Work out the finished part from the listing and answer in its coordinate system (mm). Face numbers are marked on the shaded views. A direction names the side the tool comes from. Give positions to 0.01 mm unless a question says otherwise; leave off trailing zeros. Write each loop counter-clockwise with the first axis right and the second up, starting at its lowest first coordinate (ties: lowest second). Pieces come first, ordered by that corner, then holes. Notation, with made-up numbers: (7.25, 80.5) -> (32.25, 80.5) arc R19 ccw to (32.25, 89.5) -> close; hole circle Ø9 at (-13, 29). An arc over 180 degrees is marked (long way). Use a Markdown table: item, result. Add a question column.
Q1. Section A-A, the plane z = -5.5 is taken. Give the vertices of the cut face in (x, y), plus the area to 3 significant figures.
Q2. For the marked faces 5, 6 and 7, determine the directions among +Z, -Z, +X, -X, +Y, -Y from which every point of the face is accessible in a straight line to the end or side of a thin tool.
Q3. For a pull along X with two mould halves and no side action, classify the marked faces 1, 2, 3 and 4 as pulls with the +X half, pulls with the -X half, needs draft (parallel to the pull), parting line crosses it, or undercut.
Q4. Section D-D, the plane z = 1.5 is taken. Give the vertices of the cut face in (x, y), plus the area to 3 significant figures.
Q5. Section B-B, the plane x = -1.5 is taken. Give the vertices of the cut face in (y, z).
Q6. Consider line 1 (Z direction, x = 0, y = -1.75); line 2 (X direction, y = -5, z = 0). Determine where each line is inside the solid, lowest interval first.
Q7. Each of these flat-tipped pins is pushed along its axis until it touches: pin 1 Ø4 at (x, z) = (4, 3) entering from -Y; pin 2 Ø1 at (x, y) = (0, -4) entering from +Z. Where does it stop, or does it pass through?
Q8. Section C-C, the plane y = -5.75 is taken. Give the vertices of the cut face in (x, z).
from build123d import *
from build123d import SkipClean  # not in build123d's __all__

# Parameters (mm, degrees)
F1_DEPTH = 2.5
F4_SIZE  = 0.7
F3_W     = 2.5
F3_H     = 1.2


with BuildPart() as f1:
    # F0 (on Front) → F1 (new body)
    with BuildSketch(Plane.XZ):
        with BuildLine():
            Line((0, 4), (-9, 4))
            Line((-9, 4), (-9, 3.3))
            Line((-9, 3.3), (-8.3, 3.3))
            Line((-8.3, 3.3), (-8.3, 2.6))
            Line((-8.3, 2.6), (-9, 2.6))
            Line((-9, 2.6), (-9, 1.9))
            Line((-9, 1.9), (-8.3, 1.9))
            Line((-8.3, 1.9), (-8.3, 1.2))
            Line((-8.3, 1.2), (-9, 1.2))
            Line((-9, 1.2), (-9, 0.5))
            Line((-9, 0.5), (-8.3, 0.5))
            Line((-8.3, 0.5), (-8.3, -0.2))
            Line((-8.3, -0.2), (-9, -0.2))
            Line((-9, -0.2), (-9, -7))
            Line((-9, -7), (-7.8, -7))
            Line((-7.8, -7), (-7.8, -2.900873477))
            add(Edge.make_bspline(
                [(-7.8, -2.900873477), (-7.8, -1.685574969), (-7.1826716424, -0.1281665724), (-4.9759016066, 0.6847768295), (-3.5267368498, -0.4819738014), (-3.0814464759, -1.4369020899)],
                knots=[0, 0, 0, 0, 0.3572792207, 0.6508868549, 1, 1, 1, 1], degree=3))
            ThreePointArc((-3.0814464759, -1.4369020899), (-1.8268186684, -2.8675309158), (0, -3.4))
            Line((0, -3.4), (0, -2.4))
            ThreePointArc((0, -2.4), (-2.4, 0), (0, 2.4))
            Line((0, 2.4), (0, 4))
        make_face()
    extrude(amount=F1_DEPTH)

    # F2: F1 across plane


with BuildPart() as f1_1:
    add(f1.part, clean=False)
    with SkipClean():  # cleaning this boolean's faces spoils the solid; the shape is the same uncleaned
        add(f1.part.mirror(Plane.YZ), clean=False)

    # F4
    f4_edges = [f1_1.edges().sort_by_distance(p)[0] for p in [
        (-9, -2.5, -3.6),
        (9, -2.5, -3.6),
        (-9, -2.5, 3.65),
        (-9, -2.5, 2.25),
        (-9, -2.5, 0.85),
        (9, -2.5, 3.65),
        (9, -2.5, 2.25),
        (9, -2.5, 0.85),
    ]]
    chamfer(f4_edges, length=F4_SIZE)

    # F3 (on Right) → F5 (revolve)
    with BuildSketch(Plane.YZ):
        Polygon((-2.5, 1.2), (-2.5, 2.4), (-5.3, 2.4), (-5.3, 1.9), (-6.3, 1.9), (-6.3, 2.4), (-6.8, 2.4), (-6.8, 1.2), align=None)
        with Locations((-1.25, 1.8)):
            Rectangle(F3_W, F3_H)
    revolve(axis=Axis((0, -3.9747959284, 0), (0, -1, 0)))


solid = f1_1.part
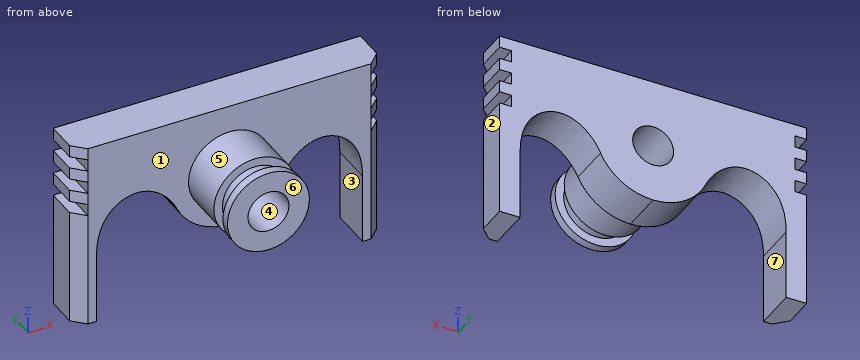
Result set:
| question | item | result |
|---|---|---|
| 1 | outline | (-9, -1.8) -> (-8.3, -2.5) -> (-7.8, -2.5) -> (-7.8, 0) -> (-9, 0) -> close; (7.8, -2.5) -> (8.3, -2.5) -> (9, -1.8) -> (9, 0) -> (7.8, 0) -> close |
| 1 | area | 5.51 mm2 |
| 2 | face 5 | -Y |
| 2 | face 6 | +Z, -Z, +X, -X, -Y |
| 2 | face 7 | -Z, +Y, -Y |
| 3 | face 1 | needs draft |
| 3 | face 2 | pulls with the +X half |
| 3 | face 3 | undercut |
| 3 | face 4 | undercut |
| 4 | outline | (-8.3, -2.5) -> (-1.87, -2.5) -> (-1.87, -5.3) -> (-1.17, -5.3) -> (-1.17, -6.3) -> (-1.87, -6.3) -> (-1.87, -6.8) -> (1.87, -6.8) -> (1.87, -6.3) -> (1.17, -6.3) -> (1.17, -5.3) -> (1.87, -5.3) -> (1.87, -2.5) -> (8.3, -2.5) -> (8.3, 0) -> (-8.3, 0) -> close |
| 4 | area | 56.2 mm2 |
| 5 | outline | (-6.8, -1.87) -> (-6.3, -1.87) -> (-6.3, -1.17) -> (-5.3, -1.17) -> (-5.3, -1.87) -> (-2.5, -1.87) -> (-2.5, -3.05) -> (0, -3.05) -> (0, 4) -> (-2.5, 4) -> (-2.5, 1.87) -> (-5.3, 1.87) -> (-5.3, 1.17) -> (-6.3, 1.17) -> (-6.3, 1.87) -> (-6.8, 1.87) -> close |
| 6 | line 1 | z = -3.4 to -1.2, 1.2 to 4 |
| 6 | line 2 | x = -2.4 to -1.2, 1.2 to 2.4 |
| 7 | pin 1 | stops at y = -2.5 |
| 7 | pin 2 | stops at z = 2.4 |
| 8 | outline | circle Ø3.8 at (0, 0); hole circle Ø2.4 at (0, 0) |
